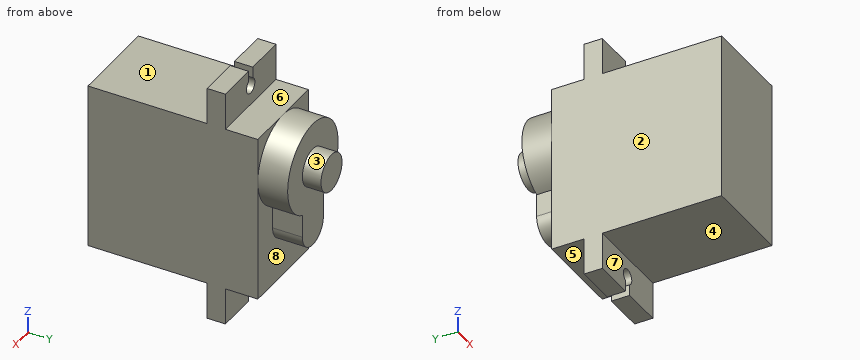
```python
from build123d import *

# Parameters (mm, degrees)
EXTRUSION1_DEPTH = 12
EXTRUSION2_DEPTH = 12.6
EXTRUSION3_DEPTH = 4
SKETCH4_R        = 2.5
EXTRUSION4_DEPTH = 2.5


with BuildPart() as part:
    # Sketch1 → Extrusion1 (new body)
    with BuildSketch(Plane.YZ):
        Polygon((0, 0), (0, 11.25), (16, 11.25), (16, 16.2), (18.45, 16.2), (18.45, 11.25), (22.8, 11.25), (22.8, 0), (22.8, -11.25), (18.45, -11.25), (18.45, -16.2), (16, -16.2), (16, -11.25), (0, -11.25), align=None)
    extrude(amount=EXTRUSION1_DEPTH)

    # Sketch2 → Extrusion2 (cut)
    with BuildSketch(Plane(origin=(0, 18.45, 0), x_dir=(-1, 0, 0), z_dir=(0, 1, 0))):
        with BuildLine():
            Line((-6.5, -14.716025404), (-6.5, -16.2))
            Line((-6.5, -16.2), (-5.5, -16.2))
            Line((-5.5, -16.2), (-5.5, -14.716025404))
            ThreePointArc((-5.5, -14.716025404), (-6, -12.85), (-6.5, -14.716025404))
        make_face()
        with BuildLine():
            Line((-6.5, 14.716025404), (-6.5, 16.2))
            Line((-6.5, 16.2), (-5.5, 16.2))
            Line((-5.5, 16.2), (-5.5, 14.716025404))
            ThreePointArc((-5.5, 14.716025404), (-6, 12.85), (-6.5, 14.716025404))
        make_face()
    extrude(amount=-EXTRUSION2_DEPTH, mode=Mode.SUBTRACT)

    # Sketch3 → Extrusion3 (add)
    with BuildSketch(Plane(origin=(0, 22.8, 0), x_dir=(-1, 0, 0), z_dir=(0, 1, 0))):
        with BuildLine():
            Line((-8.5, -0.204356057), (-8.5, -3.25))
            ThreePointArc((-8.5, -3.25), (-6, -5.75), (-3.5, -3.25))
            Line((-3.5, -3.25), (-3.5, -0.204356057))
            ThreePointArc((-3.5, -0.204356057), (-6, 11.25), (-8.5, -0.204356057))
        make_face()
    extrude(amount=EXTRUSION3_DEPTH)

    # Sketch4 → Extrusion4 (add)
    with BuildSketch(Plane(origin=(0, 26.8, 11.25), x_dir=(1, 0, 0), z_dir=(0, 1, 0))):
        with Locations((6, 6)):
            Circle(SKETCH4_R)
    extrude(amount=EXTRUSION4_DEPTH)


solid = part.part
```
Check sheet for the modelled part. Datum: model origin and axes. Units: mm. Face numbers are marked on the shaded views. A direction names the side the tool comes from. Coordinates: 2 decimals unless noted, no trailing zeros. Write each loop counter-clockwise with the first axis right and the second up, starting at its lowest first coordinate (ties: lowest second). Pieces come first, ordered by that corner, then holes. Notation, with made-up numbers: (62.25, 77) -> (120.25, 77) arc R18 cw to (120.25, 86) -> close; hole circle Ø1 at (-13, 37). An arc over 180 degrees is marked (long way). Use a Markdown table: item, result.
1. Tool access check on the marked faces 1, 2, 3, 4 and 5. Record the directions out of +Z, -Z, +X, -X, +Y, -Y that give a thin tool (end or side, any length) a straight path to the whole face; none if there is none.
Reported:
| item | result |
|---|---|
| face 1 | +Z, +X, -X, -Y |
| face 2 | +Z, -Z, -X, +Y, -Y |
| face 3 | +Y |
| face 4 | -Z, +X, -X, -Y |
| face 5 | -Z, +X, -X, +Y |
2. Go/stop test with flat-tipped pins: pin 1 Ø3 at (x, z) = (10.5, 7.5) entering from +Y; pin 2 Ø2.5 at (x, z) = (8.5, -14.5) entering from -Y; pin 3 Ø1.3 at (x, y) = (5, 20) entering from -Z; pin 4 Ø1.8 at (x, z) = (6, -13.85) entering from -Y. Record where each tip stops, or that it passes through.
Reported:
| item | result |
|---|---|
| pin 1 | stops at y = 26.8 |
| pin 2 | stops at y = 16 |
| pin 3 | stops at z = -11.25 |
| pin 4 | passes through |
3. Release check for a two-part mould opening along Y. For the marked faces 6, 7 and 8 record: pulls with the +Y half, pulls with the -Y half, needs draft (parallel to the pull), parting line crosses it, or undercut.
Reported:
| item | result |
|---|---|
| face 6 | needs draft |
| face 7 | pulls with the -Y half |
| face 8 | pulls with the +Y half |
4. Sectioned sample at B-B (z = -1). Enter the section's corners in (x, y).
Reported:
| item | result |
|---|---|
| outline | (0, 0) -> (12, 0) -> (12, 22.8) -> (8.5, 22.8) -> (8.5, 26.8) -> (3.5, 26.8) -> (3.5, 22.8) -> (0, 22.8) -> close |
5. Sectioned sample at C-C (x = 4.5). Enter the section's corners in (y, z), plus the area to 3 significant figures.
Reported:
| item | result |
|---|---|
| outline | (0, -11.25) -> (16, -11.25) -> (16, -16.2) -> (18.45, -16.2) -> (18.45, -11.25) -> (22.8, -11.25) -> (22.8, -5.25) -> (26.8, -5.25) -> (26.8, 3.25) -> (29.3, 3.25) -> (29.3, 7.25) -> (26.8, 7.25) -> (26.8, 11.06) -> (22.8, 11.06) -> (22.8, 11.25) -> (18.45, 11.25) -> (18.45, 16.2) -> (16, 16.2) -> (16, 11.25) -> (0, 11.25) -> close |
| area | 612 mm2 |
6. Sectioned sample at D-D (y = 5.75). Enter the section's corners in (x, z), plus the area to 3 significant figures.
Reported:
| item | result |
|---|---|
| outline | (0, -11.25) -> (12, -11.25) -> (12, 11.25) -> (0, 11.25) -> close |
| area | 270 mm2 |
7. Sectioned sample at A-A (z = -13.85). Enter the section's corners in (x, y), plus the area to 3 significant figures.
Reported:
| item | result |
|---|---|
| outline | (0, 16) -> (5, 16) -> (5, 18.45) -> (0, 18.45) -> close; (7, 16) -> (12, 16) -> (12, 18.45) -> (7, 18.45) -> close |
| area | 24.5 mm2 |
8. Scan lines: line 1 along Z through (x, y) = (11.25, 21); line 2 along Z through (x, y) = (6, 17.4); line 3 along Y through (x, z) = (3.25, -4). Record each from-to range of solid material in increasing order.
Reported:
| item | result |
|---|---|
| line 1 | z = -11.25 to 11.25 |
| line 2 | z = -12.85 to 12.85 |
| line 3 | y = 0 to 22.8 |
